Design review of the part built by this model. Coordinates are the model's own, in mm. Give positions to 0.01 mm unless a question says otherwise; leave off trailing zeros. Write each loop counter-clockwise with the first axis right and the second up, starting at its lowest first coordinate (ties: lowest second). Pieces come first, ordered by that corner, then holes.
```python
from build123d import *

# Parameters (mm, degrees)
SKETCH1_R           = 24.477436685
BOSS_EXTRUDE1_DEPTH = 3.175
BOSS_EXTRUDE2_START = 1.27
BOSS_EXTRUDE2_DEPTH = 1.27


with BuildPart() as part:
    # Sketch1 → Boss-Extrude1 (new body)
    with BuildSketch(Plane.XZ):
        Circle(SKETCH1_R)
    extrude(amount=BOSS_EXTRUDE1_DEPTH)

    # Sketch2 → Boss-Extrude2 (add)
    with BuildSketch(Plane(origin=(0, 0, 0), x_dir=(1, 0, 0), z_dir=(0, 1, 0)).offset(BOSS_EXTRUDE2_START)):
        with BuildLine():
            Line((1.5875, 24.425903267), (1.5875, 22.838403267))
            Line((1.5875, 22.838403267), (-1.5875, 22.838403267))
            Line((-1.5875, 22.838403267), (-1.5875, 24.425903267))
            ThreePointArc((-1.5875, 24.425903267), (0, 24.477436685), (1.5875, 24.425903267))
        make_face()
        with BuildLine():
            Line((-1.5875, -24.425903267), (-1.5875, -22.838403267))
            Line((-1.5875, -22.838403267), (1.5875, -22.838403267))
            Line((1.5875, -22.838403267), (1.5875, -24.425903267))
            ThreePointArc((1.5875, -24.425903267), (0, -24.477436685), (-1.5875, -24.425903267))
        make_face()
    extrude(amount=-BOSS_EXTRUDE2_DEPTH)


solid = part.part
```
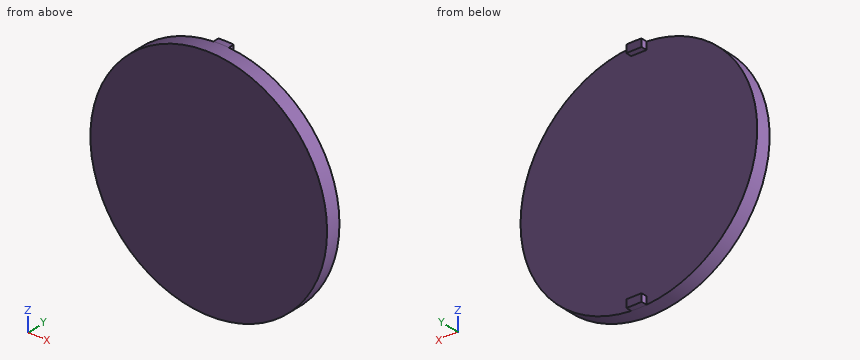
(1) To check wall thickness, follow L1, parallel to Y at x = 6.5, z = 17.5 (3 decimals); L2, parallel to Z at x = 19, y = -2.25; L3, parallel to Z at x = -2.5, y = -0.3. State the ranges of each line that lie inside material, in increasing order.
Resolved:
L1: y = -3.175 to 0
L2: z = -15.43 to 15.43
L3: z = -24.35 to 24.35
(2) Consider section C-C, the plane y = -1.6. Give the boundary of the cut face in (x, z).
Resolved:
outline: circle Ø48.95 at (0, 0)
(3) Consider section A-A, the plane x = 0. Give the boundary of the cut face in (y, z) (3 decimals).
Resolved:
outline: (-3.175, -24.477) - (1.27, -24.477) - (1.27, -22.838) - (0, -22.838) - (0, 22.838) - (1.27, 22.838) - (1.27, 24.477) - (-3.175, 24.477) - close
(4) Consider section B-B, the plane z = 0. Give the boundary of the cut face in (x, y) (3 decimals), then the cut area to 3 significant figures.
Resolved:
outline: (-24.477, -3.175) - (24.477, -3.175) - (24.477, 0) - (-24.477, 0) - close
area: 155 mm2
(5) Consider section D-D, the plane x = -18. Give the boundary of the cut face in (y, z) (1 decimal).
Resolved:
outline: (-3.2, -16.6) - (0, -16.6) - (0, 16.6) - (-3.2, 16.6) - close
(6) Clearance check with flat-ended pins moving along their axes: P1, Ø6, axis at x = -5.5, z = 18.5, coming from the +Y side; P2, Ø1, axis at x = 15.5, y = -1.5, coming from the -Z side; P3, Ø1.5, axis at x = 14.5, y = 0, coming from the +Z side. State where each tip first meets the part, or that it passes through.
Resolved:
P1: stops at y = 0
P2: stops at z = -19.34
P3: stops at z = 20.25
